Verification items for this drawing (mm, ordinates from the low corner). A direction names the side the tool comes from. Round coordinates to 2 decimals unless told otherwise and drop trailing zeros. Loops run counter-clockwise (first coordinate to the right, second up) from the corner with the lowest first, then second, coordinate; pieces in that order, holes last. Notation, with made-up numbers: M 67.5,38 L 122.5,38 A19 ccw 122.5,56 Z; hole C 6,6.25 d2. An arc over 180 degrees is marked long. Use one line per item in the form item = value. Start each with the question number.
1. Cross-section at D-D (y = 1.25). Record the boundary of the cut face in (x, z), then the cut area to 3 significant figures.
2. Go/stop test with flat-tipped pins: pin 1 (4 mm diameter, centred on x = 5, y = 3, fed in from -Z); pin 2 (1.4 mm diameter, centred on y = 2, z = 32, fed in from +X); pin 3 (1.5 mm diameter, centred on x = 7, y = 9.5, fed in from -Z) (1 decimal). Record where each tip stops, or that it passes through.
3. Draft check along Z on the marked faces 1, 2, 3 and 4. Enter one of: pulls with the +Z half, pulls with the -Z half, needs draft (parallel to the pull), parting line crosses it, or undercut.
4. Set-up check for the marked faces 5 and 6: record each of +Z, -Z, +X, -X, +Y, -Y from which the full face is reachable in a straight line by a thin tool's end or side.
5. Material ranges on line 1 (Y direction, x = 6.5, z = 27.5); line 2 (Z direction, x = 4, y = 0.5) (1 decimal); line 3 (Z direction, x = 4, y = 1.85) (1 decimal), recorded low to high.
6. Cross-section at B-B (z = 21). Record the boundary of the cut face in (x, y) (1 decimal), then the cut area to 3 significant figures.
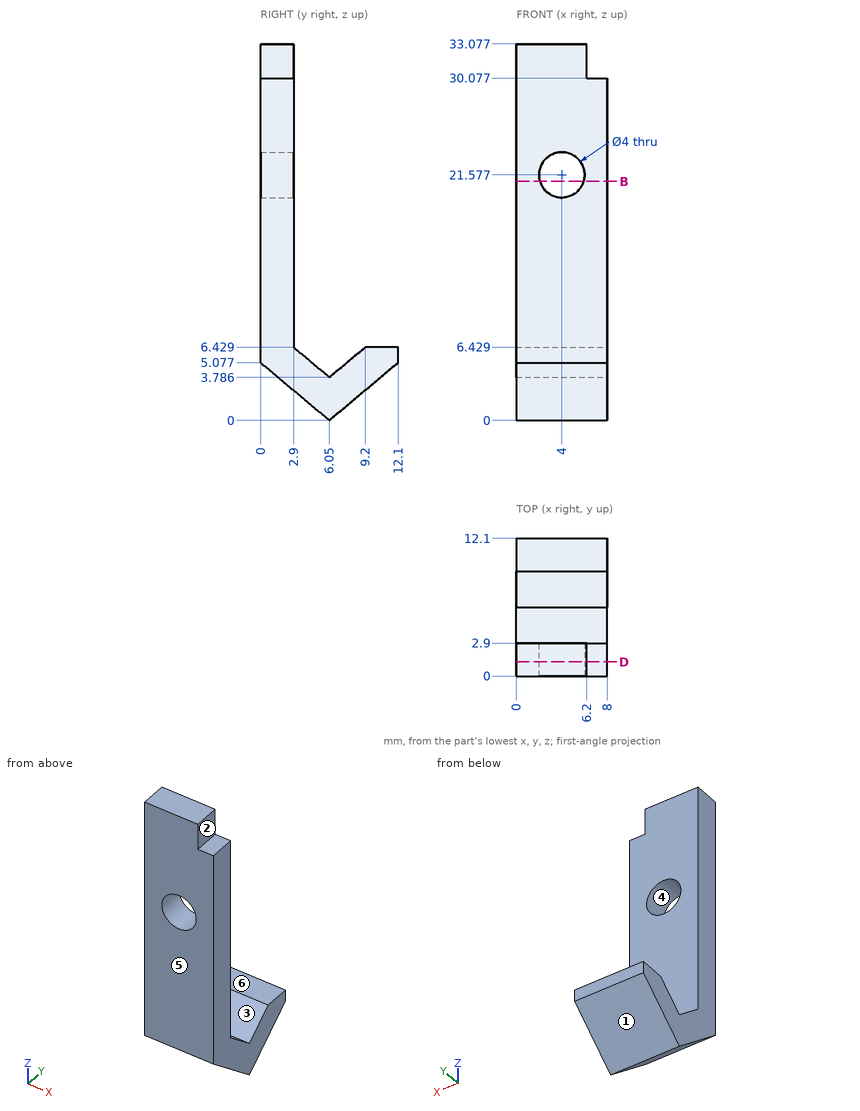
Reported:
q1.outline = M 0,4.03 L 8,4.03 L 8,30.08 L 6.2,30.08 L 6.2,33.08 L 0,33.08 Z; hole C 4,21.58 d4
q1.area = 214 mm²
q2.pin_1 = 0.88
q2.pin_2 = 6.2
q2.pin_3 = 2.3
q3.face_1 = pulls with the -Z half
q3.face_2 = needs draft
q3.face_3 = pulls with the +Z half
q3.face_4 = undercut
q4.face_5 = +Z, -Z, +X, -X, -Y
q4.face_6 = +Z, +X, -X, +Y
q5.line_1 = 0 to 2.9
q5.line_2 = 4.7 to 19.6, 23.6 to 33.1
q5.line_3 = 3.5 to 19.6, 23.6 to 33.1
q6.outline = M 0,0 L 2.1,0 L 2.1,2.9 L 0,2.9 Z; M 5.9,0 L 8,0 L 8,2.9 L 5.9,2.9 Z
q6.area = 12.1 mm²
